from build123d import *

# Parameters (mm, degrees)
EXTRUDE_1_DEPTH     = 5.5
SKETCH_2_W          = 5.5
SKETCH_2_H          = 10
CUT_EXTRUDE_1_DEPTH = 127.924442345


with BuildPart() as part:
    # ｽｹｯﾁ1 → ﾎﾞｽ - 押し出し1 (new body)
    with BuildSketch(Plane.XY):
        with BuildLine():
            Line((-10, -21.817424229), (-10, -125))
            Line((-10, -125), (10, -125))
            Line((10, -125), (10, -21.817424229))
            ThreePointArc((10, -21.817424229), (16.156067067, -17.747718076), (20.784609691, -12))
            ThreePointArc((20.784609691, -12), (19.320508076, -6.535898385), (13.856406461, -8))
            ThreePointArc((13.856406461, -8), (0, -16), (-13.856406461, -8))
            ThreePointArc((-13.856406461, -8), (-19.320508076, -6.535898385), (-20.784609691, -12))
            ThreePointArc((-20.784609691, -12), (-16.156067067, -17.747718076), (-10, -21.817424229))
        make_face()
    extrude(amount=EXTRUDE_1_DEPTH)

    # ｽｹｯﾁ2 → ｶｯﾄ - 押し出し1 (cut, through all)
    with BuildSketch(Plane.XY.offset(5.5)):
        with Locations((-7.25, -90)):
            Rectangle(SKETCH_2_W, SKETCH_2_H)
        with Locations((-7.25, -110)):
            Rectangle(SKETCH_2_W, SKETCH_2_H)
        with Locations((-7.25, -70)):
            Rectangle(SKETCH_2_W, SKETCH_2_H)
        with Locations((-7.25, -50)):
            Rectangle(SKETCH_2_W, SKETCH_2_H)
        with Locations((-7.25, -30)):
            Rectangle(SKETCH_2_W, SKETCH_2_H)
        with Locations((7.25, -110)):
            Rectangle(SKETCH_2_W, SKETCH_2_H)
        with Locations((7.25, -90)):
            Rectangle(SKETCH_2_W, SKETCH_2_H)
        with Locations((7.25, -70)):
            Rectangle(SKETCH_2_W, SKETCH_2_H)
        with Locations((7.25, -50)):
            Rectangle(SKETCH_2_W, SKETCH_2_H)
        with Locations((7.25, -30)):
            Rectangle(SKETCH_2_W, SKETCH_2_H)
    extrude(amount=-CUT_EXTRUDE_1_DEPTH, mode=Mode.SUBTRACT)


solid = part.part
Model file for the job. Use its own axes, mm. A direction names the side the tool comes from. Give positions to 0.01 mm unless a question says otherwise; leave off trailing zeros. Write each loop counter-clockwise with the first axis right and the second up, starting at its lowest first coordinate (ties: lowest second). Pieces come first, ordered by that corner, then holes. Notation, with made-up numbers: (35, 4) -> (94, 4) arc R21 ccw to (94, 35) -> close; hole circle Ø1 at (48, 23.25). An arc over 180 degrees is marked (long way). Write item = value, one per line.
(1) Probe line 1 along Y through (x, z) = (-8, 5.05); line 2 along X through (y, z) = (-58.5, 0.3); line 3 along Y through (x, z) = (5.5, 5.3). List the from-to ranges inside material, lowest first.
Determined:
line_1 = -125 to -115, -105 to -95, -85 to -75, -65 to -55, -45 to -35, -25 to -13.86
line_2 = -10 to 10
line_3 = -125 to -115, -105 to -95, -85 to -75, -65 to -55, -45 to -35, -25 to -15.02
(2) Flat gauge pins, fed straight in: P1, Ø1.6, axis at x = -8, z = 1.5, coming from the +Y side; P2, Ø1.5, axis at x = 16, z = 4, coming from the -Y side; P3, Ø3, axis at y = -120, z = 3.5, coming from the -X side. Where does each tip first touch, or does it go through?
Determined:
P1 = -13.36
P2 = -18.53
P3 = -10
(3) Slice it at C-C, the plane x = 18.5. Give the cut face in (y, z).
Determined:
outline = (-15.29, 0) -> (-6.18, 0) -> (-6.18, 5.5) -> (-15.29, 5.5) -> close
(4) Tool access for faces 1 (the face through (7, -85, 3)), 2 (the face through (-10, -60, 3)), 3 (the face through (-7, -55, 3)), 4 (the face through (10, -120, 3)): list every direction of +Z, -Z, +X, -X, +Y, -Y with a clear straight run to the whole face (end or side of a thin tool).
Determined:
face_1 = +Z, -Z, +X
face_2 = +Z, -Z, -X, -Y
face_3 = +Z, -Z, -X
face_4 = +Z, -Z, +X, -Y
(5) Slice it at B-B, the plane y = -100. Give the cut face in (x, z).
Determined:
outline = (-10, 0) -> (10, 0) -> (10, 5.5) -> (-10, 5.5) -> close
(6) Slice it at A-A, the plane y = -10. Give the cut face in (x, z), then the cut area to 3 significant figures.
Determined:
outline = (-21.32, 0) -> (-12.49, 0) -> (-12.49, 5.5) -> (-21.32, 5.5) -> close; (12.49, 0) -> (21.32, 0) -> (21.32, 5.5) -> (12.49, 5.5) -> close
area = 97.1 mm2
(7) Mould opens along Y. For faces 5 (the face through (-4.5, -70, 3)), 6 (the face through (10, -80, 3)), 7 (the face through (0, -16, 3)) say: released by +Y, released by -Y, zero draft, split by the parting line, or undercut.
Determined:
face_5 = undercut
face_6 = zero draft
face_7 = released by +Y
